Build history of the part. All positions in model axes, mm. Round coordinates to 2 decimals unless told otherwise and drop trailing zeros. Loops run counter-clockwise (first coordinate to the right, second up) from the corner with the lowest first, then second, coordinate; pieces in that order, holes last. Notation, with made-up numbers: (52.5, -26.75) -> (78.5, -26.75) arc R11 ccw to (78.5, -9.75) -> close; hole circle Ø6 at (-6, 2.25). An arc over 180 degrees is marked (long way). Put each result on its own line as item: value. Start each with the question number.
Item 1: Cut at C-C, the plane z = 161. List the corners of the cut face in (x, y), plus the area to 3 significant figures.
Item 2: Flat gauge pin, fed straight in: pin 1 Ø8.5 at (x, z) = (0, 161.925) entering from +Y. Where does the tip first touch, or does it go through?
Item 3: Cut at A-A, the plane x = 0. List the corners of the cut face in (y, z).
Item 4: Cut at D-D, the plane z = 134. List the corners of the cut face in (x, y).
Item 5: Drill centre lines: probe 1 along Z at (x, y) = (12, 0.15); probe 2 along X at (y, z) = (-0.15, 163); probe 3 along X at (y, z) = (0, 137). Where is each one in solid material? Low to high. Write a range as [from, to].
Item 6: Pull direction X, two halves, no side cores. Call faces 1 (the cylindrical face through (-1.216, 0.011, 164.858)), 2 (the flat face through (1, -0.794, 68)), 3 (the flat face through (42.5, 0, 137.6)): +X half, -X half, draft (parallel to the pull), parting line (faces both ways), or undercut.
```python
from build123d import *

# Parameters (mm, degrees)
BOSS_EXTRUDE1_DEPTH = 0.79375
FILLET1_R           = 12.7
CUT_EXTRUDE1_REACH  = 190.806
SKETCH2_R           = 3.175


with BuildPart() as part:
    # Sketch1 → Boss-Extrude1 (new, symmetric)
    with BuildSketch(Plane(origin=(0, 0, 0), x_dir=(1, 0, 0), z_dir=(0, 1, 0))):
        Polygon((-63.5, 0), (63.5, 0), (63.5, -101.6), (19.05, -177.8), (-19.05, -177.8), (-63.5, -101.6), align=None)
    extrude(amount=BOSS_EXTRUDE1_DEPTH, both=True)

    # Fillet1
    fillet1_edges = [part.edges().sort_by_distance(p)[0] for p in [
        (19.05, 0, 177.8),
        (-19.05, 0, 177.8),
        (-63.5, 0, 101.6),
        (63.5, 0, 101.6),
    ]]
    fillet(fillet1_edges, radius=FILLET1_R)

    # Sketch2 → Cut-Extrude1 (cut, up to next)
    with BuildSketch(Plane(origin=(0, 0.79375, 0), x_dir=(1, 0, 0), z_dir=(0, 1, 0)), mode=Mode.PRIVATE) as cut_extrude1_sk1:
        with Locations(Location((0, -161.925, 0), (0, 0, 270))):
            Circle(SKETCH2_R)
    cut_extrude1_tool1 = extrude(cut_extrude1_sk1.sketch, amount=-CUT_EXTRUDE1_REACH, mode=Mode.PRIVATE) & part.part
    add(cut_extrude1_tool1.solids().sort_by_distance((0, 0.79375, 161.925))[0], mode=Mode.SUBTRACT)


solid = part.part
```
Reply:
1. outline: (-28.85, -0.79) -> (-3.04, -0.79) -> (-3.04, 0.79) -> (-28.85, 0.79) -> close; (3.04, -0.79) -> (28.85, -0.79) -> (28.85, 0.79) -> (3.04, 0.79) -> close
1. area: 82.0 mm^2
2. pin 1: stops at y = 0.79
3. outline: (-0.79, 0) -> (0.79, 0) -> (0.79, 158.75) -> (-0.79, 158.75) -> close; (-0.79, 165.1) -> (0.79, 165.1) -> (0.79, 177.8) -> (-0.79, 177.8) -> close
4. outline: (-44.6, -0.79) -> (44.6, -0.79) -> (44.6, 0.79) -> (-44.6, 0.79) -> close
5. probe 1: z = [0, 177.8]
5. probe 2: x = [-27.68, -2.99], [2.99, 27.68]
5. probe 3: x = [-42.85, 42.85]
6. face 1: undercut
6. face 2: draft
6. face 3: +X half
